Autodesk Fusion 360 part; units mm, degrees
sketch "Sketch1" plane through (0, 0, 0) normal (0, 1, 0) x (1, 0, 0)
  line L0 (26.7, -27.05) -> (-26.7, -27.05)
  line L1 (-26.7, -27.05) -> (-26.7, 27.05)
  line L2 (-26.7, 27.05) -> (26.7, 27.05)
  line L3 (26.7, 27.05) -> (26.7, -27.05)
  line L4 (26.7, -27.05) -> (-26.7, 27.05) construction
  line L5 (-26.7, -27.05) -> (26.7, 27.05) construction
  line L6 (-27.7, -28.05) -> (-27.7, 28.05)
  line L7 (-27.7, 28.05) -> (27.7, 28.05)
  line L8 (27.7, 28.05) -> (27.7, -28.05)
  line L9 (27.7, -28.05) -> (-27.7, -28.05)
  dimension "d1" = 53.4
  dimension "d2" = 54.1
  dimension "d3" = -1
extrude "Extrude2" add sketch "Sketch1" along normal blind 1 contours L0 L1 L2 L3 makes body 1
extrude "Extrude1" add sketch "Sketch1" along normal blind 10 separate body makes body 2
sketch "Sketch2" plane through (-27.7, 0, 0) normal (-1, 0, 0) x (0, 0, 1)
  line L0 (-28.05, 0) -> (28.05, 0)
  line L1 (28.05, 0) -> (28.05, 10)
  line L2 (28.05, 10) -> (-28.05, 10)
  line L3 (-28.05, 10) -> (-28.05, 0)
  line L4 (-28.05, 5) -> (-6.05, 5)
  line L5 (-13, 0) -> (-13, 1)
  line L6 (-6.05, 1) -> (-17.05, 1)
  line L7 (-17.05, 1) -> (-17.05, 10)
  line L8 (-17.05, 10) -> (-6.05, 10)
  line L9 (-6.05, 10) -> (-6.05, 1)
  dimension "d8" = 22
  dimension "d9" = 11
extrude "Extrude3" cut sketch "Sketch2" against normal blind 16 contours L4 L6 L7 L9 | L2 L4 L7 L8 L9 bodies 2
sketch "Sketch3" plane through (0, 0, -28.05) normal (0, 0, -1) x (-1, 0, 0)
  line L0 (-27.7, 0) -> (27.7, 0)
  line L1 (27.7, 0) -> (27.7, 10)
  line L2 (27.7, 10) -> (-27.7, 10)
  line L3 (-27.7, 10) -> (-27.7, 0)
  line L4 (27.7, 5) -> (25.7, 5)
  line L5 (-27.7, 5) -> (-25.7, 5)
  line L6 (-23, 0) -> (-23, 1)
  line L7 (-25.7, 1) -> (-18.7, 1)
  line L8 (-18.7, 1) -> (-18.7, 10)
  line L9 (-18.7, 10) -> (-25.7, 10)
  line L10 (-25.7, 10) -> (-25.7, 1)
  line L11 (25.7, 1) -> (18.7, 1)
  line L12 (18.7, 1) -> (18.7, 10)
  line L13 (18.7, 10) -> (25.7, 10)
  line L14 (25.7, 10) -> (25.7, 1)
  dimension "d12" = 2
  dimension "d13" = 2
  dimension "d14" = 1
  dimension "d15" = 7
  dimension "d16" = 7
extrude "Extrude4" cut sketch "Sketch3" against normal blind 23 contours L2 L7 L8 L9 L10 | L2 L11 L12 L13 L14 bodies 2
sketch "Sketch4" plane through (0, 0, 0) normal (0, 1, 0) x (1, 0, 0)
  line L0 (-18.7, 28.05) -> (-13.7, 28.05)
  line L1 (-13.7, 28.05) -> (-13.7, 30.05)
  line L2 (-13.7, 30.05) -> (-7.7, 30.05)
  line L3 (-13.7, 28.05) -> (-13.7, 27.05)
  line L4 (-7.7, 27.05) -> (-13.7, 27.05)
  line L5 (-13.7, 27.05) -> (-13.7, 30.05)
  line L6 (-13.7, 30.05) -> (-7.7, 30.05)
  line L7 (-7.7, 30.05) -> (-7.7, 27.05)
  line L8 (-14.7, 26.05) -> (-14.7, 31.05)
  line L9 (-14.7, 31.05) -> (-6.7, 31.05)
  line L10 (-6.7, 31.05) -> (-6.7, 26.05)
  line L11 (-6.7, 26.05) -> (-14.7, 26.05)
  line L12 (-14.7, 28.05) -> (-13.7, 28.05)
  line L13 (-7.7, 28.05) -> (-6.7, 28.05)
  line L14 (-13.7, 28.05) -> (-7.7, 28.05)
  dimension "d19" = 5
  dimension "d20" = 2
  dimension "d21" = 6
  dimension "d22" = 1
  dimension "d23" = -1
extrude "Extrude6" add sketch "Sketch4" along normal blind 10 contours L0 L1 L2 L5 L6 L7 L8 L9 L10 L12 L13 bodies 2
extrude "Extrude5" add sketch "Sketch4" along normal blind 1 contours L1 L2 L5 L6 L7 L14 bodies 2
sketch "Sketch5" plane through (0, 10, 0) normal (0, 1, 0) x (-1, 0, 0)
  line L0 (7.7, -28.05) -> (13.7, -28.05)
  line L1 (13.7, -28.05) -> (13.7, -30.05)
  line L2 (13.7, -30.05) -> (7.7, -30.05)
  line L3 (7.7, -30.05) -> (7.7, -28.05)
  line L4 (6.7, -28.05) -> (6.7, -31.05)
  line L5 (6.7, -31.05) -> (14.7, -31.05)
  line L6 (14.7, -31.05) -> (14.7, -28.05)
  line L7 (14.7, -28.05) -> (18.7, -28.05)
  line L8 (18.7, -28.05) -> (18.7, -27.05)
  line L9 (18.7, -27.05) -> (-18.7, -27.05)
  line L10 (-18.7, -27.05) -> (-18.7, -28.05)
  line L11 (-18.7, -28.05) -> (6.7, -28.05)
  line L12 (13.7, -28.05) -> (7.7, -28.05)
  line L13 (7.7, -28.05) -> (7.7, -27.05)
  line L14 (7.7, -27.05) -> (13.7, -27.05)
  line L15 (13.7, -27.05) -> (13.7, -28.05)
extrude "Extrude7" cut sketch "Sketch5" against normal blind 9 contours L0 L9 L12 L13 L14 L15 bodies 2
sketch "Sketch6" plane through (-27.7, 0, 0) normal (-1, 0, 0) x (0, 0, 1)
  line L0 (-6.05, 10) -> (-6.05, 1)
  line L1 (-6.05, 1) -> (-17.05, 1)
  line L2 (-17.05, 1) -> (-17.05, 10)
  line L3 (-17.05, 10) -> (-28.05, 10)
  line L4 (-28.05, 10) -> (-28.05, 0)
  line L5 (-28.05, 0) -> (28.05, 0)
  line L6 (28.05, 0) -> (28.05, 10)
  line L7 (28.05, 10) -> (-6.05, 10)
  line L8 (28.05, 5) -> (20.05, 5)
  line L9 (21, 0) -> (21, 1)
  line L10 (20.05, 1) -> (9.05, 1)
  line L11 (9.05, 1) -> (9.05, 10.929)
  line L12 (9.05, 10.929) -> (20.05, 10.929)
  line L13 (20.05, 10.929) -> (20.05, 1)
  dimension "d30" = 8
  dimension "d31" = 11
extrude "Extrude8" cut sketch "Sketch6" against normal blind 9 contours L7 L11 L12 L13 | L7 L10 L11 L13 bodies 2
combine "Combine1" operation add target body 1 tool bodies 2
sketch "Sketch7" plane through (0, 0, -27.05) normal (0, 0, 1) x (1, 0, 0)
  line L0 (-7.7, 1) -> (18.7, 1)
  line L1 (18.7, 1) -> (18.7, 10)
  line L2 (18.7, 10) -> (-7.7, 10)
  line L3 (-7.7, 10) -> (-7.7, 1)
  line L4 (-7.7, 10) -> (2.3, 10)
  line L5 (2.3, 10) -> (2.3, 1)
  line L6 (2.3, 1) -> (-7.7, 1)
  line L7 (-7.7, 1) -> (-7.7, 10)
  dimension "d34" = 10
extrude "Extrude9" cut sketch "Sketch7" against normal blind 3 contours L0 L2 L3 L4 L5 L6 L7 bodies 1
sketch "Sketch8" plane through (0, 0, 0) normal (0, 1, 0) x (1, 0, 0)
extrude "Extrude10" add 1 faces at (-6.7, 3.6667, -30.7167) along direction (1, 0, 0) blind 9 on bodies 1 bodies 1
sketch "Sketch9" plane through (0, 0, -28.05) normal (0, 0, -1) x (-1, 0, 0)
  line L0 (-2.3, 0) -> (-2.3, 1)
  line L1 (-2.3, 1) -> (-2.3, 10)
  line L2 (-2.3, 10) -> (-18.7, 10)
  line L3 (-18.7, 10) -> (-18.7, 1)
  line L4 (-18.7, 1) -> (-25.7, 1)
  line L5 (-25.7, 1) -> (-25.7, 10)
  line L6 (-25.7, 10) -> (-27.7, 10)
  line L7 (-27.7, 10) -> (-27.7, 0)
  line L8 (-27.7, 0) -> (-2.3, 0)
  line L9 (-2.3, 10) -> (-3.3, 10)
  line L10 (-3.3, 10) -> (-3.3, 0)
  line L11 (-3.3, 0) -> (-2.3, 0)
  line L12 (-2.3, 0) -> (-2.3, 10)
  dimension "d39" = 1
extrude "Extrude11" add sketch "Sketch9" along normal blind 3 contours L0 L1 L2 L8 L9 L10 L11 L12 bodies 1
fillet "Fillet1" radius 2.5 4 edges at (-14.7, 5, -28.05) (-14.7, 5, -31.05) (3.3, 5, -28.05) (3.3, 5, -31.05) on bodies 1
fillet "Fillet2" radius 2 4 edges at (-27.7, 5, 28.05) (27.7, 5, 28.05) (-27.7, 5, -28.05) (27.7, 5, -28.05) on bodies 1
Verification items for the finished model (mm, model axes). A direction names the side the tool comes from. Round coordinates to 2 decimals unless told otherwise and drop trailing zeros. Loops run counter-clockwise (first coordinate to the right, second up) from the corner with the lowest first, then second, coordinate; pieces in that order, holes last. Notation, with made-up numbers: (37.25, 53.5) - (60.25, 53.5) arc R31 ccw to (60.25, 77.5) - close; hole circle Ø9 at (4, 12). An arc over 180 degrees is marked (long way). Use a Markdown table: item, result. Add a question column.
1. Thickness scan on probe 1 along X at (y, z) = (3.75, -19.5); probe 2 along Z at (x, y) = (-5.5, 5.75); probe 3 along Z at (x, y) = (13, 5.5). Record the ranges inside material, lowest first. Write a range as [from, to].
2. Section check C-C, the plane z = 6. Record the boundary of the cut face in (x, y), plus the area to 3 significant figures.
3. Section check D-D, the plane z = 17. Record the boundary of the cut face in (x, y), plus the area to 3 significant figures.
4. Access from +Z, -Z, +X, -X, +Y, -Y to the whole of each face (thin tool, end or side, straight path). Record for faces 4 (the face through (2.3, 5, -29)), 5 (the face through (-18, 3, -28.05)), 6 (the face through (13, 5, -28.05)).
5. Section check B-B, the plane y = 8.5. Give the number of separate pieces and of enclosed holes in the cut face, plus the area to 3 significant figures.
6. Release check for a two-part mould opening along Z. For faces 1 (the face through (-6, 5, -31.05)), 2 (the face through (-1, 1, -1)), 3 (the face through (27.1, 5.07, 27.48)) record: released by +Z, released by -Z, zero draft, split by the parting line, or undercut.
7. Gauge pin test, flat ends, axial feed: pin 1 (2 mm diameter, centred on x = -1.5, z = 11, fed in from +Y); pin 2 (2.5 mm diameter, centred on y = 7, z = -29, fed in from +X); pin 3 (0.8 mm diameter, centred on y = 7.5, z = -27.5, fed in from +X). Record the tip position at first contact, or that the pin passes through.
8. Section check A-A, the plane x = 16. Record the boundary of the cut face in (y, z), plus the area to 3 significant figures.
Checks:
| question | item | result |
|---|---|---|
| 1 | probe 1 | x = [-27.7, -26.7], [26.7, 27.7] |
| 1 | probe 2 | z = [-31.05, -30.05], [27.05, 28.05] |
| 1 | probe 3 | z = [-28.05, -27.05], [27.05, 28.05] |
| 2 | outline | (-27.7, 0) - (27.7, 0) - (27.7, 10) - (26.7, 10) - (26.7, 1) - (-26.7, 1) - (-26.7, 10) - (-27.7, 10) - close |
| 2 | area | 73.4 mm^2 |
| 3 | outline | (-27.7, 0) - (27.7, 0) - (27.7, 10) - (26.7, 10) - (26.7, 1) - (-27.7, 1) - close |
| 3 | area | 64.4 mm^2 |
| 4 | face 4 | +Y |
| 4 | face 5 | -Z, -X, +Y, -Y |
| 4 | face 6 | -Z, +X, +Y, -Y |
| 5 | separate pieces | 4 |
| 5 | enclosed holes | 0 |
| 5 | area | 187 mm^2 |
| 6 | face 1 | released by -Z |
| 6 | face 2 | undercut |
| 6 | face 3 | released by +Z |
| 7 | pin 1 | stops at y = 1 |
| 7 | pin 2 | stops at x = 26.75 |
| 7 | pin 3 | stops at x = 27.4 |
| 8 | outline | (0, -28.05) - (10, -28.05) - (10, -27.05) - (1, -27.05) - (1, 27.05) - (10, 27.05) - (10, 28.05) - (0, 28.05) - close |
| 8 | area | 74.1 mm^2 |
